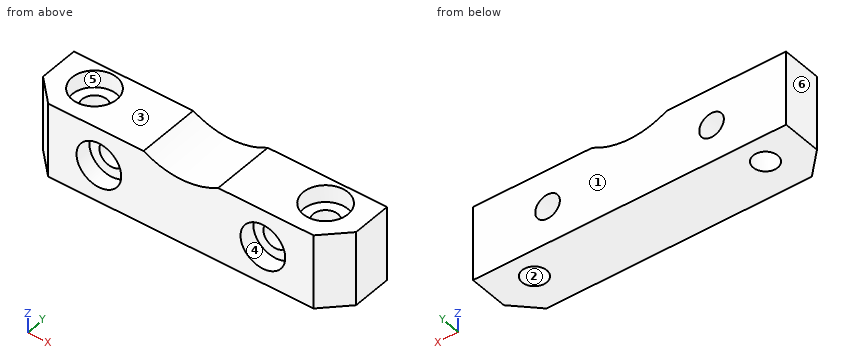
Autodesk Inventor part; units mm, degrees
ref_plane "YZ Plane" through (0, 0, 0) normal (1, 0, 0) x (0, 1, 0)
ref_plane "XZ Plane" through (0, 0, 0) normal (0, 1, 0) x (-1, 0, 0)
ref_plane "XY Plane" through (0, 0, 0) normal (0, 0, 1) x (1, 0, 0)
sketch "草圖1" plane through (0, 0, 0) normal (0, 0, 1) x (1, 0, 0)
  line L0 (-29.4, 0) -> (29.4, 0)
  line L1 (0, -5.95) -> (0, 5.95)
  line L2 (-21, 4.25) -> (21, 4.25)
  line L3 (21, 4.25) -> (21, -4.25)
  line L4 (21, -4.25) -> (-21, -4.25)
  line L5 (-21, -4.25) -> (-21, 4.25)
  point P0 (0, 0)
  dimension "d0" = 8.5
  dimension "d1" = 42
extrude "擠出1" add sketch "草圖1" along normal blind 10
sketch "草圖2" plane through (-21, -4.25, 0) normal (0, -1, 0) x (1, 0, 0)
  line L0 (0, 0) -> (42, 0)
  line L1 (42, 0) -> (42, 10)
  line L2 (0, 10) -> (42, 10)
  line L3 (0, 0) -> (0, 10)
  circle A0 centre (10, 5) radius 4
  circle A1 centre (10, 5) radius 3
  circle A2 centre (10, 5) radius 1.65
  line L4 (21, 0) -> (21, -1.5889)
  circle A3 centre (32, 5) radius 4
  circle A4 centre (32, 5) radius 3
  circle A5 centre (32, 5) radius 1.65
  dimension "d4" = 6
  dimension "d5" = 3.3
  dimension "d6" = 10
  dimension "d29" = 5
extrude "擠出2" cut sketch "草圖2" against normal blind 10 contours A2 | A5
extrude "擠出3" cut sketch "草圖2" against normal blind 2.2 contours A1 | A4
sketch "草圖3" plane through (0, 0, 10) normal (0, 0, 1) x (1, 0, 0)
  line L0 (-21, -4.25) -> (21, -4.25)
  line L1 (21, -4.25) -> (21, 4.25)
  line L2 (21, 4.25) -> (-21, 4.25)
  line L3 (-21, 4.25) -> (-21, -4.25)
  line L4 (-17.8, -4.25) -> (-21, -1.05)
  line L5 (0, 4.25) -> (0, 6.2817)
  line L6 (17.8, -4.25) -> (21, -1.05)
  line L7 (17.8, -4.25) -> (22.3255, -4.25) construction
  circle A0 centre (-15.5, 0.75) radius 1.65
  circle A1 centre (-15.5, 0.75) radius 3
  circle A2 centre (15.5, 0.75) radius 1.65
  circle A3 centre (15.5, 0.75) radius 3
  point P0 (0, 0)
  dimension "d11" = 3.2
  dimension "d12" = 45
  dimension "d13" = 45
  dimension "d14" = 3.2
  dimension "d15" = 3.3
  dimension "d16" = 6
  dimension "d17" = 5.5
  dimension "d24" = 3.5
extrude "擠出4" cut sketch "草圖3" against normal up to surface (10 mm away) contours L3 L4 L0 | L6 L1 L0 | A0 | A2
extrude "擠出6" cut sketch "草圖3" against normal blind 2.3 contours A1 | A3
sketch "草圖4" plane through (-17.8, -4.25, 0) normal (0, -1, 0) x (1, 0, 0)
  line L0 (0, 10) -> (0, 0)
  line L1 (0, 0) -> (35.6, 0)
  line L2 (35.6, 0) -> (35.6, 10)
  line L3 (0, 10) -> (35.6, 10)
  circle A0 centre (28.8, 5) radius 3
  circle A1 centre (6.8, 5) radius 3
  arc A2 (12.8, 10) -> (22.8, 10) centre (17.8, 18.6603) ccw
  line L4 (17.8, 10) -> (17.8, 8.9301)
  point P0 (17.8, 0)
  dimension "d25" = 10
  dimension "d26" = 10
extrude "擠出7" cut sketch "草圖4" against normal up to surface (8.5 mm away) contours L3 A2
equation "\"d27\" = d25"
properties part number "y_motor_lock_bottom1_3D 列印"
CAD build for the part. Positions are in the model's coordinates, mm. Face numbers are marked on the shaded views. A direction names the side the tool comes from. Coordinates: 2 decimals unless noted, no trailing zeros. Write each loop counter-clockwise with the first axis right and the second up, starting at its lowest first coordinate (ties: lowest second). Pieces come first, ordered by that corner, then holes. Notation, with made-up numbers: (19.25, 61) -> (50.25, 61) arc R31 ccw to (50.25, 88) -> close; hole circle Ø1 at (5, -23.5). An arc over 180 degrees is marked (long way). Return JSON: item names as keys, results as strings. Group by question number.
Q1. Cut at B-B, the plane x = -11. Give the cut face in (y, z).
Q2. Pull direction Y, two halves, no side cores. Call the marked faces 1, 2 and 3: released by +Y, released by -Y, zero draft, split by the parting line, or undercut.
Q3. Which spindle directions (+Z, -Z, +X, -X, +Y, -Y) get a long thin tool onto all of the face, cutting with end or side? Do the marked faces 4, 5 and 6. Say none if no direction does.
Q4. Cut at C-C, the plane z = 6.25. Give the cut face in (x, y).
Q5. Cut at A-A, the plane y = 0.75. Give the cut face in (x, z).
Q6. Flat gauge pins, fed straight in: pin 1 (1.8 mm diameter, centred on x = -17, y = -0.5, fed in from +Z); pin 2 (5 mm diameter, centred on x = 11, z = 5, fed in from -Y); pin 3 (1.5 mm diameter, centred on y = -2, z = 1.5, fed in from -X). Where does each tip first touch, or does it go through?
Q7. Drill centre lines: line 1 (Z direction, x = -11, y = -3.4); line 2 (Z direction, x = -11, y = 0.5); line 3 (X direction, y = -1.5, z = 6). Where is each one in solid material? Low to high.
Q8. Cut at D-D, the plane x = -15.5. Give the cut face in (y, z), then the cut area to 3 significant figures.
Returned:
{
 "1": {"outline": "(-4.25, 0) -> (4.25, 0) -> (4.25, 3.35) -> (-2.05, 3.35) -> (-2.05, 2) -> (-4.25, 2) -> close; (-4.25, 8) -> (-2.05, 8) -> (-2.05, 6.65) -> (4.25, 6.65) -> (4.25, 10) -> (-4.25, 10) -> close"},
 "2": {"face 1": "released by +Y", "face 2": "undercut", "face 3": "zero draft"},
 "3": {"face 4": "-Y", "face 5": "+Z", "face 6": "+Z, -Z, -X, +Y, -Y"},
 "4": {"outline": "(-21, -1.05) -> (-17.8, -4.25) -> (-13.73, -4.25) -> (-13.73, -2.05) -> (-12.08, -2.05) -> (-12.08, 4.25) -> (-21, 4.25) -> close; (-9.92, -2.05) -> (-8.27, -2.05) -> (-8.27, -4.25) -> (8.27, -4.25) -> (8.27, -2.05) -> (9.92, -2.05) -> (9.92, 4.25) -> (-9.92, 4.25) -> close; (12.08, -2.05) -> (13.73, -2.05) -> (13.73, -4.25) -> (17.8, -4.25) -> (21, -1.05) -> (21, 4.25) -> (12.08, 4.25) -> close; hole circle Ø3.3 at (-15.5, 0.75); hole circle Ø3.3 at (15.5, 0.75)"},
 "5": {"outline": "(-21, 0) -> (-17.15, 0) -> (-17.15, 7.7) -> (-18.5, 7.7) -> (-18.5, 10) -> (-21, 10) -> close; (-13.85, 0) -> (13.85, 0) -> (13.85, 7.7) -> (12.5, 7.7) -> (12.5, 10) -> (5, 10) arc R10 cw to (-5, 10) -> (-12.5, 10) -> (-12.5, 7.7) -> (-13.85, 7.7) -> close; (17.15, 0) -> (21, 0) -> (21, 10) -> (18.5, 10) -> (18.5, 7.7) -> (17.15, 7.7) -> close; hole circle Ø3.3 at (-11, 5); hole circle Ø3.3 at (11, 5)"},
 "6": {"pin 1": "stops at z = 7.7", "pin 2": "stops at y = -2.05", "pin 3": "stops at x = -20.8"},
 "7": {"line 1": "z = 0 to 2, 8 to 10", "line 2": "z = 0 to 3.35, 6.65 to 10", "line 3": "x = -20.55 to -12.31, -9.69 to 9.69, 12.31 to 20.55"},
 "8": {"outline": "(-4.25, 0) -> (-0.9, 0) -> (-0.9, 7.7) -> (-2.25, 7.7) -> (-2.25, 10) -> (-4.25, 10) -> close; (2.4, 0) -> (4.25, 0) -> (4.25, 10) -> (3.75, 10) -> (3.75, 7.7) -> (2.4, 7.7) -> close", "area": "45.8 mm2"}
}
